Work out the finished part from the listing and answer in its coordinate system (mm). A direction names the side the tool comes from. Round coordinates to 2 decimals unless told otherwise and drop trailing zeros. Write each loop counter-clockwise with the first axis right and the second up, starting at its lowest first coordinate (ties: lowest second). Pieces come first, ordered by that corner, then holes. Notation, with made-up numbers: (68, 33.25) -> (116, 33.25) arc R23 cw to (116, 55.25) -> close; hole circle Ø7 at (61.25, 65). An arc over 180 degrees is marked (long way). One line per question, with ' | ' between items. Start each with the question number.
```python
from build123d import *

# Parameters (mm, degrees)
SKETCH_1_R          = 20
EXTRUDE_1_DEPTH     = 12
SKETCH_3_R          = 14
CUT_EXTRUDE_3_DEPTH = 8
SKETCH_4_R          = 7
CUT_EXTRUDE_4_DEPTH = 31.724582991


with BuildPart() as part:
    # Эскиз1 → Вытянуть1 (new body)
    with BuildSketch(Plane(origin=(0, 0, 0), x_dir=(1, 0, 0), z_dir=(0, 1, 0))):
        with Locations(Location((0, 0, 0), (0, 0, 270))):
            Circle(SKETCH_1_R)
    extrude(amount=EXTRUDE_1_DEPTH)

    # Эскиз3 → Вытянуть3 (cut)
    with BuildSketch(Plane.XZ):
        with Locations(Location((0, 0, 0), (0, 0, 270))):
            Circle(SKETCH_3_R)
    extrude(amount=-CUT_EXTRUDE_3_DEPTH, mode=Mode.SUBTRACT)

    # Эскиз4 → Вытянуть4 (cut, through all)
    with BuildSketch(Plane(origin=(0, 12, 0), x_dir=(1, 0, 0), z_dir=(0, 1, 0))):
        with Locations(Location((0, 0, 0), (0, 0, 270))):
            Circle(SKETCH_4_R)
    extrude(amount=-CUT_EXTRUDE_4_DEPTH, mode=Mode.SUBTRACT)


solid = part.part
```
(1) A cutting plane is placed at C-C, the plane y = 10. Determine the outline of the cut face in (x, z), then the cut area to 3 significant figures.
(2) The mould has two halves that part along X. Classify faces 1 (the cylindrical face through (-19.524, 5.916, -4.336)), 2 (the cylindrical face through (-13.67, 3.94, 3.03)), 3 (the cylindrical face through (-6.834, 10.028, -1.517)), 4 (the flat face through (14, 0, 4)): +X half, -X half, draft (parallel to the pull), parting line (faces both ways), or undercut.
(3) Given pin 1 Ø18 at (x, z) = (0, 0) entering from -Y; pin 2 Ø1.5 at (y, z) = (4, 14.5) entering from +X; pin 3 Ø1.5 at (x, y) = (-15, 5.5) entering from +Z, each flat-ended and moving along its own axis, determine where each tip first touches the part or whether it passes through.
(4) For faces 5 (the flat face through (3.3, 8, 6.4)), 6 (the flat face through (0, 12, 9)), determine the directions among +Z, -Z, +X, -X, +Y, -Y from which every point of the face is accessible in a straight line to the end or side of a thin tool.
(5) Consider L1, parallel to X at y = 2, z = 0; L2, parallel to X at y = 11.15, z = 0; L3, parallel to Y at x = 1.5, z = -9. Determine where each line is inside the solid, lowest interval first.
(6) A cutting plane is placed at D-D, the plane x = -11.5. Determine the outline of the cut face in (y, z), then the cut area to 3 significant figures.
(7) A cutting plane is placed at B-B, the plane x = 0. Determine the outline of the cut face in (y, z), then the cut area to 3 significant figures.
(8) A cutting plane is placed at A-A, the plane z = 0. Determine the outline of the cut face in (x, y), then the cut area to 3 significant figures.
Returned:
1) outline: circle Ø40 at (0, 0); hole circle Ø14 at (0, 0) | area: 1,100 mm2
2) face 1: parting line | face 2: undercut | face 3: undercut | face 4: draft
3) pin 1: y = 8 | pin 2: x = 14.52 | pin 3: z = 14.03
4) face 5: -Y | face 6: +Z, -Z, +X, -X, +Y
5) L1: -20 to -14, 14 to 20 | L2: -20 to -7, 7 to 20 | L3: 8 to 12
6) outline: (0, -16.36) -> (12, -16.36) -> (12, 16.36) -> (0, 16.36) -> (0, 7.98) -> (8, 7.98) -> (8, -7.98) -> (0, -7.98) -> close | area: 265 mm2
7) outline: (0, -20) -> (12, -20) -> (12, -7) -> (8, -7) -> (8, -14) -> (0, -14) -> close; (0, 14) -> (8, 14) -> (8, 7) -> (12, 7) -> (12, 20) -> (0, 20) -> close | area: 200 mm2
8) outline: (-20, 0) -> (-14, 0) -> (-14, 8) -> (-7, 8) -> (-7, 12) -> (-20, 12) -> close; (7, 8) -> (14, 8) -> (14, 0) -> (20, 0) -> (20, 12) -> (7, 12) -> close | area: 200 mm2
